Drawing for the job (mm, zero at the part's lowest x, y, z). Coordinates: 2 decimals unless noted, no trailing zeros. Write each loop counter-clockwise with the first axis right and the second up, starting at its lowest first coordinate (ties: lowest second). Pieces come first, ordered by that corner, then holes. Notation, with made-up numbers: (-29.75, 78) -> (5.25, 78) arc R8 cw to (5.25, 88) -> close; hole circle Ø1 at (66, 30.5). An arc over 180 degrees is marked (long way). Write each question's results on one line, items separated by ' | '. Start each with the question number.
Q1. Drop a flat-ended pin along its axis: pin 1 Ø1.5 at (y, z) = (110.5, 2.5) entering from -X. Give the stop position or say it passes through.
Q2. Drill centre lines: line 1 (X direction, y = 14, z = 2.3) (1 decimal); line 2 (X direction, y = 21, z = 1.3); line 3 (X direction, y = 94, z = 1.9). Where is each one in solid material? Low to high.
Q3. Saw through at D-D on x = 7. Give the cut face in (y, z) (1 decimal).
Q4. Saw through at A-A on x = 19. Give the cut face in (y, z) (1 decimal), and give its area (3 significant figures).
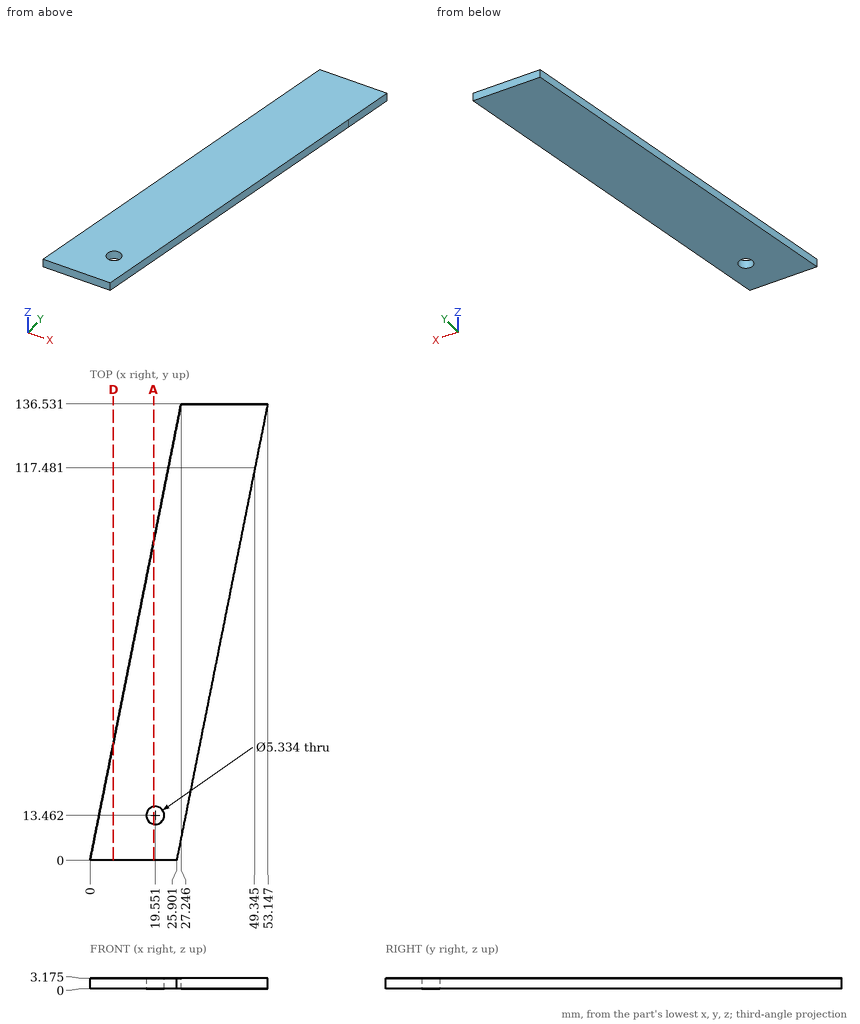
Returned:
1) pin 1: stops at x = 21.9
2) line 1: x = 2.8 to 16.9, 22.2 to 28.7 | line 2: x = 4.19 to 30.09 | line 3: x = 18.76 to 44.66
3) outline: (0, 0) -> (35.1, 0) -> (35.1, 3.2) -> (0, 3.2) -> close
4) outline: (0, 0) -> (10.9, 0) -> (10.9, 3.2) -> (0, 3.2) -> close; (16.1, 0) -> (95.2, 0) -> (95.2, 3.2) -> (16.1, 3.2) -> close | area: 286 mm2
